Geometry: final body of the model. Coordinates: model frame, mm. Face numbers are marked on the shaded views. A direction names the side the tool comes from. Give positions to 0.01 mm unless a question says otherwise; leave off trailing zeros. Write each loop counter-clockwise with the first axis right and the second up, starting at its lowest first coordinate (ties: lowest second). Pieces come first, ordered by that corner, then holes.
Q1. Cut plane C-C on x = -20.32. Count the separate pieces of the cut face and the enclosed holes in it, plus the area to 3 significant figures.
Q2. Reachability of the marked faces 4, 5, 6, 7 and 8 from +Z, -Z, +X, -X, +Y, -Y: full face, straight path, thin tool, end or side. Return the list, or none.
Q3. Draft query along Z for the marked faces 1, 2 and 3. Return one class per face: pulls with the +Z half, pulls with the -Z half, needs draft (parallel to the pull), parting line crosses it, or undercut.
Q4. Pin query (flat end, axial travel): pin 1 (6 mm diameter, centred on x = 0, y = 1, fed in from +Z); pin 2 (1.3 mm diameter, centred on x = -20, z = -5, fed in from -Y); pin 3 (8 mm diameter, centred on y = -20.5, z = -30, fed in from -X); pin 4 (12 mm diameter, centred on y = 25.5, z = -19, fed in from -X). Return the tip coordinate at first contact, or that it passes through.
Q5. Cut plane B-B on y = 10.5. Return the cut outline in (x, z) (3 decimals), plus the area to 3 significant figures.
Q6. Line query: L1, parallel to X at y = 13.97, z = -0.6; L2, parallel to X at y = 11, z = -17.5; L3, parallel to Y at x = 20.32, z = -0.8. Output: solid intervals per line, ascending.
Q7. Cut plane D-D on z = -28. Return the cut outline in (x, y), plus the area to 3 significant figures.
Q8. Cut plane A-A on z = -12. Return the cut outline in (x, y), plus the area to 3 significant figures.
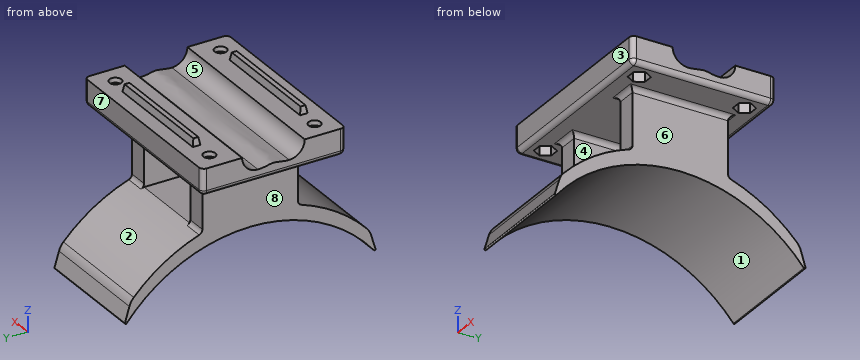
```python
from build123d import *

# Parameters (mm, degrees)
F1_W          = 50.8
F1_H          = 38.1
F2_DEPTH      = 6.985
F4_DEPTH      = 50.8
F6_DEPTH      = 15.24
F6_DEPTH_BACK = 15.24
F7_W          = 20
F7_H          = 15.9418935353
F8_DEPTH      = 25.4
F9_R          = 1.6
F10_DEPTH     = 25.4
F11_R         = 1.6
F12_DEPTH     = 5.7
F13_W         = 30.48
F13_H         = 2
F14_DEPTH     = 2
F14_TAPER     = 10
F15_F1_R      = 0.254
F15_F2_R      = 0.254
F16_R         = 5.08
F17_R         = 1.27


# Not quite as in the source:
# - two fillets or chamfers of one size are made in one step


with BuildPart() as f2:
    # F1 (on Top) → F2 (new body)
    with BuildSketch(Plane.XY):
        Rectangle(F1_W, F1_H)
    extrude(amount=-F2_DEPTH)

    # F3 (on face) → F4 (cut, through all)
    with BuildSketch(Plane.YZ.offset(25.4)):
        with BuildLine():
            add(Edge.make_bspline(
                [(-4.125, 4.125), (-2.4255892558, 4.1137489608), (-0.0276085061, 2.971292738), (2.5249406681, 4.1137612248), (4.191, 4.191)],
                knots=[0, 0, 0, 0, 0.4977710734, 1, 1, 1, 1], degree=3))
            ThreePointArc((-4.125, 4.125), (-7.0418154724, 2.9168154724), (-8.25, 0))
            ThreePointArc((-8.25, 0), (-7.0418154724, -2.9168154724), (-4.125, -4.125))
            add(Edge.make_bspline(
                [(-4.125, -4.125), (-2.9335741419, -4.2006121948), (0.4172014685, -3.0581585459), (2.1438994445, -4.2006121948), (4.191, -4.191)],
                knots=[0, 0, 0, 0, 0.497799261, 1, 1, 1, 1], degree=3))
            ThreePointArc((4.191, -4.191), (7.15448452, -2.96348452), (8.382, 0))
            ThreePointArc((8.382, 0), (7.15448452, 2.96348452), (4.191, 4.191))
        make_face()
    extrude(amount=-F4_DEPTH, mode=Mode.SUBTRACT)

    # F5 (on Right) → F6 (join, two sides)
    with BuildSketch(Plane.YZ) as f6_sk:
        with BuildLine():
            ThreePointArc((-33.655, -41.5313687512), (0, -24.985), (33.655, -41.5313687512))
            Line((33.655, -41.5313687512), (31.75, -35.2327876972))
            ThreePointArc((31.75, -35.2327876972), (23.0609926669, -27.7856916423), (12.7, -22.9268935353))
            ThreePointArc((12.7, -22.9268935353), (0, -20.985), (-12.7, -22.9268935353))
            ThreePointArc((-12.7, -22.9268935353), (-23.0609926669, -27.7856916423), (-31.75, -35.2327876972))
            Line((-31.75, -35.2327876972), (-33.655, -41.5313687512))
        make_face()
        with BuildLine():
            ThreePointArc((-12.7, -22.9268935353), (0, -20.985), (12.7, -22.9268935353))
            Line((12.7, -22.9268935353), (12.7, -6.985))
            Line((12.7, -6.985), (-12.7, -6.985))
            Line((-12.7, -6.985), (-12.7, -22.9268935353))
        make_face()
    extrude(amount=F6_DEPTH)
    extrude(f6_sk.sketch, amount=-F6_DEPTH_BACK)

    # F7 (on face) → F8 (cut)
    with BuildSketch(Plane.XZ.offset(12.7)):
        with Locations((0, -14.9559467677)):
            Rectangle(F7_W, F7_H)
    extrude(amount=-F8_DEPTH, mode=Mode.SUBTRACT)

    # F9 (on face) → F10 (cut)
    with BuildSketch(Plane(origin=(0, 0, -6.985), x_dir=(1, 0, 0), z_dir=(0, 0, -1))):
        with Locations((20.32, -13.97)):
            Circle(F9_R)
        with Locations((-20.32, -13.97)):
            Circle(F9_R)
        with Locations((-20.32, 13.97)):
            Circle(F9_R)
        with Locations((20.32, 13.97)):
            Circle(F9_R)
    extrude(amount=-F10_DEPTH, mode=Mode.SUBTRACT)

    # F11 (on face) → F12 (cut)
    with BuildSketch(Plane(origin=(0, 0, -6.985), x_dir=(1, 0, 0), z_dir=(0, 0, -1))):
        Polygon((21.645, -16.26496732), (22.97, -13.97), (21.645, -11.67503268), (18.995, -11.67503268), (17.67, -13.97), (18.995, -16.26496732), align=None)
        with Locations((20.32, -13.97)):
            Circle(F11_R, mode=Mode.SUBTRACT)
        Polygon((-18.995, -11.67503268), (-21.645, -11.67503268), (-22.97, -13.97), (-21.645, -16.26496732), (-18.995, -16.26496732), (-17.67, -13.97), align=None)
        with Locations((-20.32, -13.97)):
            Circle(F11_R, mode=Mode.SUBTRACT)
        Polygon((-18.995, 11.67503268), (-17.67, 13.97), (-18.995, 16.26496732), (-21.645, 16.26496732), (-22.97, 13.97), (-21.645, 11.67503268), align=None)
        with Locations((-20.32, 13.97)):
            Circle(F11_R, mode=Mode.SUBTRACT)
        Polygon((18.995, 11.67503268), (21.645, 11.67503268), (22.97, 13.97), (21.645, 16.26496732), (18.995, 16.26496732), (17.67, 13.97), align=None)
        with Locations((20.32, 13.97)):
            Circle(F11_R, mode=Mode.SUBTRACT)
    extrude(amount=-F12_DEPTH, mode=Mode.SUBTRACT)

    # F13 (on face) → F14 (join)
    with BuildSketch(Plane.XY):
        with Locations((0, 14.24)):
            Rectangle(F13_W, F13_H)
        with Locations((0, -14.24)):
            Rectangle(F13_W, F13_H)
    extrude(amount=F14_DEPTH, taper=F14_TAPER)

    # F15: fillet of radius 0.254 on 2 edges, made by hand

    # F15_f1
    f15_f1_edges = [f2.edges().sort_by_distance(p)[0] for p in [
        (0, -33.655, -41.5313687512),
    ]]
    fillet(f15_f1_edges, radius=F15_F1_R)

    # F15_f2
    f15_f2_edges = [f2.edges().sort_by_distance(p)[0] for p in [
        (0, 33.655, -41.5313687512),
    ]]
    fillet(f15_f2_edges, radius=F15_F2_R)

    # F16
    f16_edges = [f2.edges().sort_by_distance(p)[0] for p in [
        (0, 31.75, -35.232788),
        (0, -31.75, -35.232788),
    ]]
    fillet(f16_edges, radius=F16_R)

    # F17
    f17_edges = [f2.edges().sort_by_distance(p)[0] for p in [
        (-15.24, 0, -6.985),
        (12.62, 12.7, -22.926894),
        (-12.62, 12.7, -22.926894),
        (-12.62, 12.7, -6.985),
        (0, 19.05, -6.985),
        (25.4, 0, -6.985),
        (-25.4, 0, -6.985),
        (0, -19.05, -6.985),
        (-12.62, -12.7, -6.985),
        (-10, 0, -6.985),
        (12.62, -12.7, -6.985),
        (15.24, 0, -6.985),
        (10, 0, -6.985),
        (12.62, 12.7, -6.985),
        (-12.62, -12.7, -22.926894),
        (12.62, -12.7, -22.926894),
        (25.4, 19.05, -3.4925),
        (-25.4, 19.05, -3.4925),
        (25.4, -19.05, -3.4925),
        (-25.4, -19.05, -3.4925),
    ]]
    fillet(f17_edges, radius=F17_R)


solid = f2.part
```
Data:
1. separate pieces: 3
1. enclosed holes: 0
1. area: 145 mm2
2. face 4: +Y, -Y
2. face 5: +Z, +X, -X
2. face 6: -Z, +X, +Y, -Y
2. face 7: +Z, +X, -X, +Y
2. face 8: -Z, -X, +Y, -Y
3. face 1: pulls with the -Z half
3. face 2: undercut
3. face 3: needs draft
4. pin 1: stops at z = -3.63
4. pin 2: stops at y = -19.05
4. pin 3: stops at x = -15.24
4. pin 4: passes through
5. outline: (-25.4, -5.715) arc R1.27 ccw to (-24.13, -6.985) - (-16.51, -6.985) arc R1.27 cw to (-15.24, -8.255) - (-15.24, -26.302) - (15.24, -26.302) - (15.24, -8.255) arc R1.27 cw to (16.51, -6.985) - (24.13, -6.985) arc R1.27 ccw to (25.4, -5.715) - (25.4, 0) - (-25.4, 0) - close; hole (-10, -22.927) - (10, -22.927) - (10, -8.255) arc R1.27 ccw to (8.73, -6.985) - (-8.73, -6.985) arc R1.27 ccw to (-10, -8.255) - close
5. area: 625 mm2
6. L1: x = -25.4 to -21.92, -18.72 to 18.72, 21.92 to 25.4
6. L2: x = -15.24 to -10, 10 to 15.24
6. L3: y = -19.05 to -15.57, -12.37 to -8.17, 8.3 to 12.37, 15.57 to 19.05
7. outline: (-15.24, -23.39) - (15.24, -23.39) - (15.24, -15.72) - (-15.24, -15.72) - close; (-15.24, 15.72) - (15.24, 15.72) - (15.24, 23.39) - (-15.24, 23.39) - close
7. area: 467 mm2
8. outline: (-15.24, -12.7) - (-10, -12.7) - (-10, 12.7) - (-15.24, 12.7) - close; (10, -12.7) - (15.24, -12.7) - (15.24, 12.7) - (10, 12.7) - close
8. area: 266 mm2
